Input: part model. Units: mm. Frame: model coordinates. Round coordinates to 2 decimals unless told otherwise and drop trailing zeros. Loops run counter-clockwise (first coordinate to the right, second up) from the corner with the lowest first, then second, coordinate; pieces in that order, holes last.
(1) Line query: line 1 (Y direction, x = 44.45, z = 1.05); line 2 (Y direction, x = -8.89, z = 0.9); line 3 (X direction, y = 2, z = 1.1). Output: solid intervals per line, ascending.
(2) Cut plane B-B, the plane z = 1.25. Give the number of separate pieces and of enclosed holes in the cut face, and give its area (3 significant figures).
(3) Cut plane A-A, the plane y = 2.54. Output: boundary loops of the cut face in (x, z), and give its area (3 significant figures).
(4) Draft query along Y for faces 1 (the face through (46.66, 14, 1)), 2 (the face through (17, 0, 1)), 3 (the face through (-9.47, 28, 0.79)), 4 (the face through (17, 29.2, 1)). Return one class per face: released by +Y, released by -Y, zero draft, split by the parting line, or undercut.
(5) First-contact query: pin 1 Ø2.5 at (x, y) = (-10.16, 2.54) entering from +Z. Flat tip, straight axial feed; report the tip coordinate or a pass-through.
Autodesk Inventor part; units mm, degrees
ref_plane "YZ Plane" through (0, 0, 0) normal (1, 0, 0) x (0, 1, 0)
ref_plane "XZ Plane" through (0, 0, 0) normal (0, 1, 0) x (-1, 0, 0)
ref_plane "XY Plane" through (0, 0, 0) normal (0, 0, 1) x (1, 0, 0)
sketch "Эскиз1" plane through (0, 0, 0) normal (0, 0, 1) x (1, 0, 0)
  line L0 (-12.7, 0) -> (46.66, 0)
  line L1 (46.66, 0) -> (46.66, 29.2)
  line L2 (46.66, 29.2) -> (-12.7, 29.2)
  line L3 (-12.7, 29.2) -> (-12.7, 0)
  circle A0 centre (-8.89, 13.97) radius 0.8
  circle A1 centre (-8.89, 8.97) radius 0.8
  circle A2 centre (43.18, 8.89) radius 0.8
  circle A3 centre (43.18, 13.89) radius 0.8
  circle A4 centre (-10.16, 26.67) radius 1.5
  circle A5 centre (44.45, 26.67) radius 1.5
  circle A6 centre (44.45, 2.54) radius 1.5
  circle A7 centre (-10.16, 2.54) radius 1.5
extrude "untitled.brdКонтур" add sketch "Эскиз1" along normal blind 1.6
properties part number "untitled.brdКонтур"
Reported:
1. line 1: y = 0 to 1.04, 4.04 to 25.17, 28.17 to 29.2
1. line 2: y = 0 to 1.74, 3.34 to 8.17, 9.77 to 13.17, 14.77 to 25.87, 27.47 to 29.2
1. line 3: x = -12.7 to -11.56, -8.76 to 43.05, 45.85 to 46.66
2. separate pieces: 1
2. enclosed holes: 8
2. area: 1,700 mm2
3. outline: (-12.7, 0) - (-11.66, 0) - (-11.66, 1.6) - (-12.7, 1.6) - close; (-8.66, 0) - (42.95, 0) - (42.95, 1.6) - (-8.66, 1.6) - close; (45.95, 0) - (46.66, 0) - (46.66, 1.6) - (45.95, 1.6) - close
3. area: 85.4 mm2
4. face 1: zero draft
4. face 2: released by -Y
4. face 3: undercut
4. face 4: released by +Y
5. pin 1: passes through
